from build123d import *

# Parameters (mm, degrees)
SKETCH1_W             = 45
SKETCH1_H             = 32.5
BOSS_EXTRUDE1_DEPTH   = 17
CUT_EXTRUDE1_DEPTH    = 6.5
M3_TAPPED_HOLE1_D     = 2.5
M3_TAPPED_HOLE1_DEPTH = 10
M3_TAPPED_HOLE1_TIP   = 0.751075774


with BuildPart() as part:
    # Sketch1 → Boss-Extrude1 (new body)
    with BuildSketch(Plane(origin=(0, 0, 0), x_dir=(1, 0, 0), z_dir=(0, 1, 0))):
        Rectangle(SKETCH1_W, SKETCH1_H)
        with BuildLine():
            Line((-15.8, -9.2), (-15.8, 9.2))
            ThreePointArc((-15.8, 9.2), (-12.5, 12.5), (-9.2, 9.2))
            Line((-9.2, 9.2), (-9.2, -9.2))
            ThreePointArc((-9.2, -9.2), (-12.5, -12.5), (-15.8, -9.2))
        make_face(mode=Mode.SUBTRACT)
        with BuildLine():
            Line((9.2, -9.2), (9.2, 9.2))
            ThreePointArc((9.2, 9.2), (12.5, 12.5), (15.8, 9.2))
            Line((15.8, 9.2), (15.8, -9.2))
            ThreePointArc((15.8, -9.2), (12.5, -12.5), (9.2, -9.2))
        make_face(mode=Mode.SUBTRACT)
    extrude(amount=BOSS_EXTRUDE1_DEPTH)

    # Sketch2 → Cut-Extrude1 (cut)
    with BuildSketch(Plane(origin=(0, 17, 0), x_dir=(1, 0, 0), z_dir=(0, 1, 0))):
        with BuildLine():
            Line((18, -9.2), (18, 9.2))
            ThreePointArc((18, 9.2), (12.5, 14.7), (7, 9.2))
            Line((7, 9.2), (7, -9.2))
            ThreePointArc((7, -9.2), (12.5, -14.7), (18, -9.2))
        make_face()
        with BuildLine():
            Line((-7, -9.2), (-7, 9.2))
            ThreePointArc((-7, 9.2), (-12.5, 14.7), (-18, 9.2))
            Line((-18, 9.2), (-18, -9.2))
            ThreePointArc((-18, -9.2), (-12.5, -14.7), (-7, -9.2))
        make_face()
    extrude(amount=-CUT_EXTRUDE1_DEPTH, mode=Mode.SUBTRACT)

    # M3 Tapped Hole1
    with Locations(Plane(origin=(0, 0, -16.25), x_dir=(-1, 0, 0), z_dir=(0, 0, -1))):
        with Locations((-18.5, 5), (0, 12), (18.5, 5)):
            Hole(M3_TAPPED_HOLE1_D / 2, depth=M3_TAPPED_HOLE1_DEPTH)
            with Locations((0, 0, -(M3_TAPPED_HOLE1_DEPTH + M3_TAPPED_HOLE1_TIP / 2))):  # 118° drill point
                Cone(0, M3_TAPPED_HOLE1_D / 2, M3_TAPPED_HOLE1_TIP, mode=Mode.SUBTRACT)


solid = part.part
The model under review builds one solid part; all positions refer to its coordinate system, in mm. A direction names the side the tool comes from. Round coordinates to 2 decimals unless told otherwise and drop trailing zeros. Write each loop counter-clockwise with the first axis right and the second up, starting at its lowest first coordinate (ties: lowest second). Pieces come first, ordered by that corner, then holes. Notation, with made-up numbers: (29.25, -17) -> (49.25, -17) arc R8 ccw to (49.25, -7) -> close; hole circle Ø8 at (-28, 81). An arc over 180 degrees is marked (long way). Answer as a JSON object with one key per item and string values.
1. The part is to be moulded in two halves that separate along Z. For faces 1 (the face through (18.29, 5.07, -5.63)), 2 (the face through (0, 8, 16.25)), 3 (the face through (-15.8, 5, 0)), say which applies: pulls with the +Z half, pulls with the -Z half, needs draft (parallel to the pull), parting line crosses it, or undercut.
Results found:
{"face 1": "pulls with the -Z half", "face 2": "pulls with the +Z half", "face 3": "undercut"}
2. We need section B-B on x = 12.5. State the section outline as (y, z) points, and give its area (3 significant figures).
Results found:
{"outline": "(0, -16.25) -> (17, -16.25) -> (17, -14.7) -> (10.5, -14.7) -> (10.5, -12.5) -> (0, -12.5) -> close; (0, 12.5) -> (10.5, 12.5) -> (10.5, 14.7) -> (17, 14.7) -> (17, 16.25) -> (0, 16.25) -> close", "area": "98.9 mm^2"}
3. Clearance check with flat-ended pins moving along their axes: pin 1 (4 mm diameter, centred on x = 12.5, z = -6.5, fed in from +Y); pin 2 (3.5 mm diameter, centred on x = 10, z = -6, fed in from +Y); pin 3 (2 mm diameter, centred on x = -18.5, y = 5, fed in from -Z). State where each tip first meets the part, or that it passes through.
Results found:
{"pin 1": "passes through", "pin 2": "stops at y = 10.5", "pin 3": "stops at z = -6.1"}
4. To check wall thickness, follow line 1 along X through (y, z) = (7.5, -2); line 2 along X through (y, z) = (15.75, -9.5); line 3 along X through (y, z) = (12, -8.25). State the ranges of each line that lie inside material, in increasing order.
Results found:
{"line 1": "x = -22.5 to -15.8, -9.2 to 9.2, 15.8 to 22.5", "line 2": "x = -22.5 to -17.99, -7.01 to 7.01, 17.99 to 22.5", "line 3": "x = -22.5 to -18, -7 to -1.25, 1.25 to 7, 18 to 22.5"}
5. Machinability: for faces 4 (the face through (0, 8, -16.25)), 5 (the face through (15.8, 5, 0)), 6 (the face through (12.6, 13.8, -14.7)), which of the approach directions +Z, -Z, +X, -X, +Y, -Y give a long, thin tool a straight path to every point of the face, cutting with its end or side? Answer none if there is none.
Results found:
{"face 4": "-Z, +X, -X, +Y, -Y", "face 5": "+Y, -Y", "face 6": "+Y"}
6. We need section A-A on z = -4.5. State the section outline as (x, y) points, and give its area (3 significant figures).
Results found:
{"outline": "(-22.5, 0) -> (-15.8, 0) -> (-15.8, 10.5) -> (-18, 10.5) -> (-18, 17) -> (-22.5, 17) -> close; (-9.2, 0) -> (9.2, 0) -> (9.2, 10.5) -> (7, 10.5) -> (7, 17) -> (-7, 17) -> (-7, 10.5) -> (-9.2, 10.5) -> close; (15.8, 0) -> (22.5, 0) -> (22.5, 17) -> (18, 17) -> (18, 10.5) -> (15.8, 10.5) -> close", "area": "483 mm^2"}
7. We need section C-C on z = -11.5. State the section outline as (x, y) points, and give its area (3 significant figures).
Results found:
{"outline": "(-22.5, 0) -> (-14.87, 0) -> (-14.87, 10.5) -> (-17.5, 10.5) -> (-17.5, 17) -> (-22.5, 17) -> close; (-10.13, 0) -> (10.13, 0) -> (10.13, 10.5) -> (7.5, 10.5) -> (7.5, 17) -> (-7.5, 17) -> (-7.5, 10.5) -> (-10.13, 10.5) -> close; (14.87, 0) -> (22.5, 0) -> (22.5, 17) -> (17.5, 17) -> (17.5, 10.5) -> (14.87, 10.5) -> close; hole circle Ø2.5 at (-18.5, 5); hole circle Ø2.5 at (0, 12); hole circle Ø2.5 at (18.5, 5)", "area": "521 mm^2"}
8. We need section D-D on y = 1.5. State the section outline as (x, z) points.
Results found:
{"outline": "(-22.5, -16.25) -> (22.5, -16.25) -> (22.5, 16.25) -> (-22.5, 16.25) -> close; hole (-15.8, -9.2) arc R3.3 ccw to (-9.2, -9.2) -> (-9.2, 9.2) arc R3.3 ccw to (-15.8, 9.2) -> close; hole (9.2, -9.2) arc R3.3 ccw to (15.8, -9.2) -> (15.8, 9.2) arc R3.3 ccw to (9.2, 9.2) -> close"}
